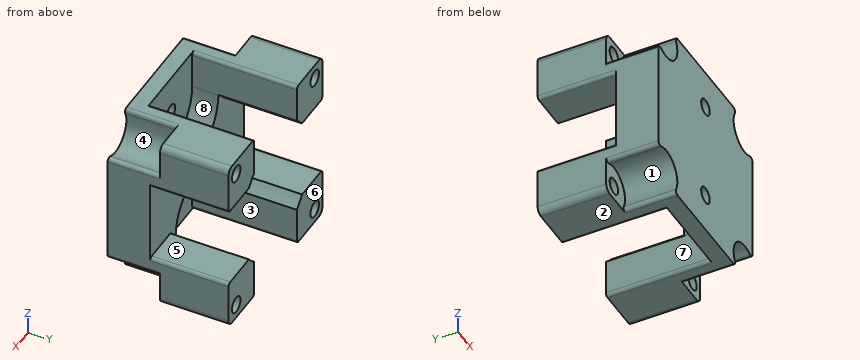
from build123d import *

# Parameters (mm, degrees)
SKETCH1_W               = 55
SKETCH1_H               = 55
BOSS_EXTRUDE1_DEPTH     = 37
SKETCH2_R               = 20
CUT_EXTRUDE1_DEPTH      = 24
SKETCH3_W               = 25
SKETCH3_H               = 55
CUT_EXTRUDE2_DEPTH      = 24
SKETCH4_W               = 55
SKETCH4_H               = 25
CUT_EXTRUDE3_DEPTH      = 24
SKETCH5_R               = 2.5
CUT_EXTRUDE4_DEPTH      = 38
SKETCH6_R               = 2.5
CUT_EXTRUDE5_DEPTH      = 38
SKETCH8_R               = 6.5
CUT_EXTRUDE6_DEPTH      = 16
CUT_EXTRUDE11_DEPTH     = 8
SKETCH16_W              = 25
SKETCH16_H              = 12
CUT_EXTRUDE12_DEPTH     = 8
SKETCH17_W              = 25
SKETCH17_H              = 12
CUT_EXTRUDE13_DEPTH     = 8
SKETCH18_R              = 2.5
CUT_EXTRUDE14_DEPTH     = 6
MIRROR5_COPY_1_SKETCH_R = 6.5
MIRROR5_COPY_1_DEPTH    = 16
FILLET2_R               = 2
FILLET3_R               = 1
FILLET4_R               = 1


with BuildPart() as part:
    # Sketch1 → Boss-Extrude1 (new body)
    with BuildSketch(Plane(origin=(0, 0, 0), x_dir=(1, 0, 0), z_dir=(0, 1, 0))):
        with Locations((27.5, 27.5)):
            Rectangle(SKETCH1_W, SKETCH1_H)
    extrude(amount=BOSS_EXTRUDE1_DEPTH)

    # Sketch2 → Cut-Extrude1 (cut)
    with BuildSketch(Plane(origin=(0, 37, 0), x_dir=(1, 0, 0), z_dir=(0, 1, 0))):
        with Locations((27.5, 27.5)):
            Circle(SKETCH2_R)
    extrude(amount=-CUT_EXTRUDE1_DEPTH, mode=Mode.SUBTRACT)

    # Sketch3 → Cut-Extrude2 (cut)
    with BuildSketch(Plane(origin=(0, 37, 0), x_dir=(1, 0, 0), z_dir=(0, 1, 0))):
        with Locations((27.5, 27.5)):
            Rectangle(SKETCH3_W, SKETCH3_H)
    cut_extrude2 = extrude(amount=-CUT_EXTRUDE2_DEPTH, mode=Mode.SUBTRACT)

    # Sketch4 → Cut-Extrude3 (cut)
    with BuildSketch(Plane(origin=(0, 37, 0), x_dir=(1, 0, 0), z_dir=(0, 1, 0))):
        with Locations((27.5, 27.5)):
            Rectangle(SKETCH4_W, SKETCH4_H)
    extrude(amount=-CUT_EXTRUDE3_DEPTH, mode=Mode.SUBTRACT)

    # Sketch5 → Cut-Extrude4 (cut, through all)
    with BuildSketch(Plane(origin=(0, 37, 0), x_dir=(1, 0, 0), z_dir=(0, 1, 0))):
        with Locations((4.5, 4.5)):
            Circle(SKETCH5_R)
    cut_extrude4 = extrude(amount=-CUT_EXTRUDE4_DEPTH, mode=Mode.SUBTRACT)

    # Sketch6 → Cut-Extrude5 (cut, through all)
    with BuildSketch(Plane(origin=(0, 37, 0), x_dir=(1, 0, 0), z_dir=(0, 1, 0))):
        with Locations((50.5, 4.5)):
            Circle(SKETCH6_R)
    cut_extrude5 = extrude(amount=-CUT_EXTRUDE5_DEPTH, mode=Mode.SUBTRACT)

    # Mirror1: Cut-Extrude4, Cut-Extrude5 across plane
    add(cut_extrude4.mirror(Plane(origin=(0, 0, -27.5), x_dir=(1, 0, 0), z_dir=(0, 0, -1))), mode=Mode.SUBTRACT)
    add(cut_extrude5.mirror(Plane(origin=(0, 0, -27.5), x_dir=(1, 0, 0), z_dir=(0, 0, -1))), mode=Mode.SUBTRACT)

    # Sketch8 → Cut-Extrude6 (cut)
    with BuildSketch(Plane.XZ):
        with Locations((50.5, -50.5)):
            Circle(SKETCH8_R)
    cut_extrude6 = extrude(amount=-CUT_EXTRUDE6_DEPTH, mode=Mode.SUBTRACT)

    # Sketch15 → Cut-Extrude11 (cut)
    with BuildSketch(Plane(origin=(0, 13, 0), x_dir=(1, 0, 0), z_dir=(0, 1, 0))):
        with BuildLine():
            ThreePointArc((24, 55), (20, 33), (40, 43))
            ThreePointArc((40, 43), (37.5, 50.5), (31, 55))
            Line((31, 55), (24, 55))
        make_face()
        with BuildLine():
            Line((24, 55), (31, 55))
            ThreePointArc((31, 55), (27.5, 55.5), (24, 55))
        make_face()
    cut_extrude11 = extrude(amount=-CUT_EXTRUDE11_DEPTH, mode=Mode.SUBTRACT)

    # Sketch16 → Cut-Extrude12 (cut)
    with BuildSketch(Plane(origin=(0, 13, 0), x_dir=(1, 0, 0), z_dir=(0, 1, 0))):
        with Locations((27.5, 49)):
            Rectangle(SKETCH16_W, SKETCH16_H)
    extrude(amount=-CUT_EXTRUDE12_DEPTH, mode=Mode.SUBTRACT)

    # Mirror2: Cut-Extrude2, Cut-Extrude11 across plane
    add(cut_extrude2.mirror(Plane(origin=(0, 0, -27.5), x_dir=(1, 0, 0), z_dir=(0, 0, -1))), mode=Mode.SUBTRACT)
    add(cut_extrude11.mirror(Plane(origin=(0, 0, -27.5), x_dir=(1, 0, 0), z_dir=(0, 0, -1))), mode=Mode.SUBTRACT)

    # Sketch17 → Cut-Extrude13 (cut)
    with BuildSketch(Plane(origin=(0, 13, 0), x_dir=(1, 0, 0), z_dir=(0, 1, 0))):
        with Locations((27.5, 6)):
            Rectangle(SKETCH17_W, SKETCH17_H)
    extrude(amount=-CUT_EXTRUDE13_DEPTH, mode=Mode.SUBTRACT)

    # Sketch18 → Cut-Extrude14 (cut, through all)
    with BuildSketch(Plane(origin=(0, 5, 0), x_dir=(1, 0, 0), z_dir=(0, 1, 0))):
        with Locations((27.5, 43)):
            Circle(SKETCH18_R)
    cut_extrude14 = extrude(amount=-CUT_EXTRUDE14_DEPTH, mode=Mode.SUBTRACT)

    # Mirror3: Cut-Extrude14 across plane
    add(cut_extrude14.mirror(Plane(origin=(0, 0, -27.5), x_dir=(1, 0, 0), z_dir=(0, 0, -1))), mode=Mode.SUBTRACT)

    # Mirror4: Cut-Extrude6 across plane
    add(cut_extrude6.mirror(Plane(origin=(27.5, 0, 0), x_dir=(0, 0, 1), z_dir=(1, 0, 0))), mode=Mode.SUBTRACT)

    # Mirror5: Cut-Extrude6 across plane
    add(cut_extrude6.mirror(Plane(origin=(0, 0, -27.5), x_dir=(1, 0, 0), z_dir=(0, 0, -1))), mode=Mode.SUBTRACT)

    # Mirror5 copy 1 sketch → Mirror5 copy 1 (cut)
    with BuildSketch(Plane(origin=(55, 0, -55), x_dir=(-1, 0, 0), z_dir=(0, -1, 0))):
        with Locations((50.5, -50.5)):
            Circle(MIRROR5_COPY_1_SKETCH_R)
    extrude(amount=-MIRROR5_COPY_1_DEPTH, mode=Mode.SUBTRACT)

    # Fillet2
    fillet2_edges = [part.edges().sort_by_distance(p)[0] for p in [
        (0, 26.5, -55),
        (55, 26.5, -55),
        (55, 26.5, 0),
        (0, 26.5, 0),
    ]]
    fillet(fillet2_edges, radius=FILLET2_R)

    # Fillet3
    fillet3_edges = [part.edges().sort_by_distance(p)[0] for p in [
        (55, 8, -45.80958424),
        (45.80958424, 8, -55),
        (0, 8, -45.80958424),
        (9.19041576, 8, -55),
        (0, 8, -9.19041576),
        (9.19041576, 8, 0),
        (45.80958424, 8, 0),
        (55, 8, -9.19041576),
    ]]
    fillet(fillet3_edges, radius=FILLET3_R)

    # Fillet4
    fillet4_edges = [part.edges().sort_by_distance(p)[0] for p in [
        (15, 21, 0),
        (40, 21, -55),
        (15, 21, -55),
        (40, 21, 0),
        (0, 25, -40),
        (55, 25, -15),
        (0, 25, -15),
        (55, 25, -40),
    ]]
    fillet(fillet4_edges, radius=FILLET4_R)


solid = part.part
Work out the finished part from the listing and answer in its coordinate system (mm). Face numbers are marked on the shaded views. A direction names the side the tool comes from. Coordinates: 2 decimals unless noted, no trailing zeros. Write each loop counter-clockwise with the first axis right and the second up, starting at its lowest first coordinate (ties: lowest second). Pieces come first, ordered by that corner, then holes. Notation, with made-up numbers: M 89,42.25 L 96,42.25 A25 ccw 96,66.25 Z; hole C 68,38.5 d2. An arc over 180 degrees is marked long. Answer as CSV lines item,"result". Start each with the question number.
Item 1: Section B-B on x = 27.5 is taken. Write down the section's boundary in (y, z), and give its area (3 significant figures).
Item 2: Section C-C on y = 30 is taken. Give the number of separate pieces and of enclosed holes in the cut face, and give its area (3 significant figures).
Item 3: Section A-A on z = -50.5 is taken. Write down the section's boundary in (x, y).
Item 4: Determine the mould class of the marked faces 1, 2 and 3 for opening direction Z: released by +Z, released by -Z, zero draft, split by the parting line, or undercut.
Item 5: Consider L1, parallel to X at y = 32, z = -4.5; L2, parallel to Z at x = 27.5, y = 2.15; L3, parallel to Z at x = 4.5, y = 27.75. Determine where each line is inside the solid, lowest interval first.
Item 6: Flat-ended cylindrical pins translate along their axes: P1, Ø1.5, axis at x = 34, z = -32.5, coming from the +Y side; P2, Ø5.5, axis at x = 47, z = -49.5, coming from the -Y side. Find the tip coordinate at first contact, or state that the pin passes through.
Item 7: Section D-D on x = 35.5 is taken. Write down the section's boundary in (y, z), and give its area (3 significant figures).
Item 8: A tool of negligible diameter and unlimited length cuts with its end or side. For the marked faces 4, 5, 6, 7 and 8, from which of +Z, -Z, +X, -X, +Y, -Y can it reach the whole face along a straight path? Write none if from no direction.
Checks:
1,outline,"M 0,-55 L 5,-55 L 5,-45.5 L 0,-45.5 Z; M 0,-40.5 L 5,-40.5 L 5,-30.5 L 13,-30.5 L 13,-24.5 L 5,-24.5 L 5,-14.5 L 0,-14.5 Z; M 0,-9.5 L 5,-9.5 L 5,0 L 0,0 Z"
1,area,"273 mm²"
2,separate pieces,"4"
2,enclosed holes,"4"
2,area,"796 mm²"
3,outline,"M 0,16 L 2,16 L 2,37 L 0,37 Z; M 7,16 L 11,16 L 11,0 L 44,0 L 44,16 L 48,16 L 48,37 L 40,37 L 40,5 L 15,5 L 15,37 L 7,37 Z; M 53,16 L 55,16 L 55,37 L 53,37 Z"
4,face 1,"undercut"
4,face 2,"released by -Z"
4,face 3,"zero draft"
5,L1,"x = 0 to 2, 7 to 15, 40 to 48, 53 to 55"
5,L2,"z = -55 to -45.5, -40.5 to -14.5, -9.5 to 0"
5,L3,"z = -55 to -53, -48 to -40, -15 to -7, -2 to 0"
6,P1,"stops at y = 13"
6,P2,"stops at y = 16"
7,outline,"M 0,-55 L 5,-55 L 5,-33.4 L 13,-33.4 L 13,-21.6 L 5,-21.6 L 5,0 L 0,0 Z"
7,area,"369 mm²"
8,face 4,"-Y"
8,face 5,"+X, -X, +Y"
8,face 6,"+Z, -Z, +X, -X, +Y"
8,face 7,"-Z, +Y"
8,face 8,"+Z, +Y"
